Autodesk Inventor part; units mm, degrees
ref_plane "YZ Plane" through (0, 0, 0) normal (1, 0, 0) x (0, 1, 0)
ref_plane "XZ Plane" through (0, 0, 0) normal (0, 1, 0) x (-1, 0, 0)
ref_plane "XY Plane" through (0, 0, 0) normal (0, 0, 1) x (1, 0, 0)
sketch "Sketch1" plane through (0, 0, 0) normal (0, 1, 0) x (-1, 0, 0)
  circle A0 centre (0, 0) radius 17
  dimension "d0" = 34
extrude "Extrusion1" add sketch "Sketch1" against normal blind 30
sketch "Sketch2" plane through (0, -30, 0) normal (0, -1, 0) x (1, 0, 0)
  circle A0 centre (0, 0) radius 17
  line L0 (0, 0) -> (0, -21) construction
  line L1 (0, 0) -> (-24, 0) construction
  line L2 (0, -21) -> (-24, -21)
  line L3 (-24, 0) -> (-24, -21)
  line L4 (0, -21) -> (24, -21)
  line L5 (24, 0) -> (24, -21)
  line L6 (0, 21) -> (-24, 21)
  line L7 (-24, 0) -> (-24, 21)
  line L8 (0, 21) -> (24, 21)
  line L9 (24, 0) -> (24, 21)
  dimension "d5" = 21
  dimension "d6" = 24
extrude "Extrusion2" add sketch "Sketch2" along normal blind 6 contours A0 | L2 L3 L7 L6 L8 L9 L5 L4
sketch "Sketch3" plane through (-24, -30, 21) normal (0, 0, 1) x (1, 0, 0)
  line L0 (0, 0) -> (48, 0)
  line L1 (48, -6) -> (0, -6)
  line L2 (3, -6) -> (45, -6)
  line L3 (45, -6) -> (45, -3)
  line L4 (45, -3) -> (3, -3)
  line L5 (3, -3) -> (3, -6)
  line L6 (24, 0) -> (24, -6) construction
  line L7 (24, -3) -> (24, -6) construction
  point P0 (24, 30)
  dimension "d9" = 3
  dimension "d11" = 42
extrude "Extrusion3" cut sketch "Sketch3" against normal through all
sketch "Sketch4" plane through (0, 0, 0) normal (0, 0, 1) x (1, 0, 0)
  line L0 (-21, -33) -> (21, -33)
  line L1 (21, -33) -> (21, -75)
  line L2 (21, -75) -> (-21, -75)
  line L3 (-21, -75) -> (-21, -33)
  line L4 (-21, -36) -> (-21, -33)
  line L5 (-21, -33) -> (21, -33)
  line L6 (21, -33) -> (21, -36)
  point P0 (0, 0)
extrude "Extrusion4" add sketch "Sketch4" along normal mid plane 90
sketch "Sketch5" plane through (0, 0, 45) normal (0, 0, 1) x (1, 0, 0)
  line L0 (21, -33) -> (-21, -33)
  line L1 (-21, -33) -> (-21, -75)
  line L2 (-21, -75) -> (21, -75)
  line L3 (21, -75) -> (21, -33)
  line L4 (-21, -33) -> (21, -75) construction
  circle A0 centre (0, -54) radius 21
  point P0 (0, 0)
extrude "Extrusion5" cut sketch "Sketch5" against normal blind 10 contours L3 A0 L0 | A0 L1 L0 | L3 L2 A0 | A0 L2 L1
move or copy body "Move Body1" bodies to move or copy 1 copy no rotation origin (0, 0, 0) rotation axis (1, 0, 0) rotation angle 90
move or copy body "Move Body2" bodies to move or copy 1 copy no rotation origin (0, 0, 0) rotation axis (0, 0, 1) rotation angle 90
move or copy body "Move Body3" bodies to move or copy 1 copy no translate (0, 0, 54)
properties part number "Wrist_Yaw"
Input: part model. Units: mm. Frame: model coordinates. A direction names the side the tool comes from. Coordinates: 2 decimals unless noted, no trailing zeros. Loops run counter-clockwise (first coordinate to the right, second up) from the corner with the lowest first, then second, coordinate; pieces in that order, holes last. Notation, with made-up numbers: M 8.25,81 L 51.25,81 A22 ccw 51.25,109 Z; hole C 41.5,7.5 d8. An arc over 180 degrees is marked long. Use a Markdown table: item, result. Add a question column.
1) Section D-D, the plane x = 18.5. Return the cut outline in (y, z), plus the area to 3 significant figures.
2) Pin query (flat end, axial travel): P1, Ø3, axis at x = -33.5, y = -11, coming from the +Z side; P2, Ø2.5, axis at x = 7, y = 22.5, coming from the -Z side; P3, Ø12.5, axis at x = -17, z = 4.5, coming from the +Y side. Return the tip coordinate at first contact, or that it passes through.
3) Section B-B, the plane z = 30. Return the cut outline in (x, y).
4) Section A-A, the plane x = 0. Return the cut outline in (y, z), plus the area to 3 significant figures.
5) Set-up query: faces 1 (the flat face through (35, 17, -17)), 2 (the cylindrical face through (14.334, -9.139, 39.21)), 3 (the flat face through (35, -17, -16)). Return all of +Z, -Z, +X, -X, +Y, -Y with unobstructed straight access to the full face (end or side cutting, diameter ignored); none if empty.
6) Section C-C, the plane y = 7. Return the cut outline in (x, z).
7) Line query: L1, parallel to Y at x = -2.5, z = 1.5; L2, parallel to Z at x = 16.5, y = 15. Output: solid intervals per line, ascending. Write a range as from..to.
Answer below:
| question | item | result |
|---|---|---|
| 1 | outline | M -24,18 L -21,18 L -21,-21 L 21,-21 L 21,18 L 24,18 L 24,24 L -24,24 Z |
| 1 | area | 1,930 mm2 |
| 2 | P1 | z = 21 |
| 2 | P2 | z = 18 |
| 2 | P3 | y = 21 |
| 3 | outline | C 0,0 d34 |
| 4 | outline | M -24,18 L -21,18 L -21,-21 L 21,-21 L 21,18 L 24,18 L 24,24 L 17,24 L 17,54 L -17,54 L -17,24 L -24,24 Z |
| 4 | area | 2,950 mm2 |
| 5 | face 1 | -Z, +X, +Y |
| 5 | face 2 | +Z |
| 5 | face 3 | -Z, +X, -Y |
| 6 | outline | M -45,-21 L 35,-21 L 35,-19.8 L 45,-19.8 L 45,19.8 L 35,19.8 L 35,21 L 21,21 L 21,24 L 15.49,24 L 15.49,54 L -15.49,54 L -15.49,24 L -21,24 L -21,21 L -45,21 Z |
| 7 | L1 | -21..21 |
| 7 | L2 | -21..24 |
